Here's how the part is built. I have some questions about the finished solid (model axes, mm). Face numbers are marked on the shaded views. A direction names the side the tool comes from. Round coordinates to 2 decimals unless told otherwise and drop trailing zeros. Write each loop counter-clockwise with the first axis right and the second up, starting at its lowest first coordinate (ties: lowest second). Pieces come first, ordered by that corner, then holes. Notation, with made-up numbers: (20.5, -10) -> (47.5, -10) arc R7 ccw to (47.5, 0) -> close; hole circle Ø5 at (36, 36). An arc over 180 degrees is marked (long way). Answer as CSV lines item,"result".
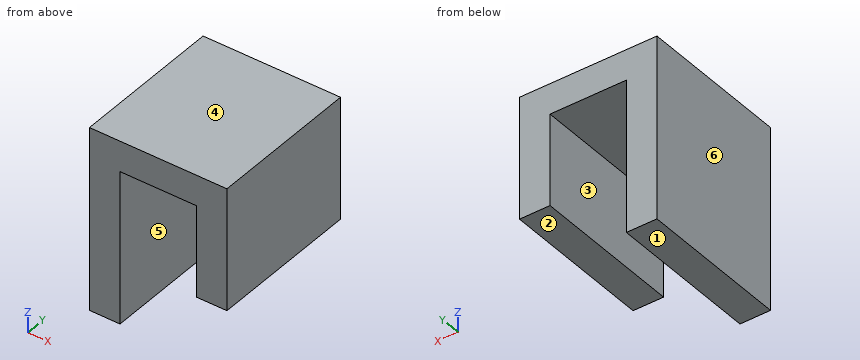
Autodesk Fusion 360 part; units mm, degrees
sketch "Sketch1" plane through (0, 0, 0) normal (0, 0, 1) x (1, 0, 0)
  line L0 (0, 0) -> (2, 0)
  line L1 (2, 0) -> (2, 10)
  line L2 (2, 10) -> (0, 10)
  line L3 (0, 10) -> (0, 0)
  dimension "d4" = 10
  dimension "d5" = 2
extrude "Extrude1" add sketch "Sketch1" along normal blind 12
sketch "Sketch2" plane through (2, 0, 0) normal (1, 0, 0) x (0, 1, 0)
  line L0 (0, 0) -> (10, 0)
  line L1 (10, 0) -> (10, 12)
  line L2 (10, 12) -> (0, 12)
  line L3 (0, 12) -> (0, 0)
  line L4 (0, 12) -> (10, 12)
  line L5 (10, 12) -> (10, 10)
  line L6 (10, 10) -> (0, 10)
  line L7 (0, 10) -> (0, 12)
  dimension "d8" = 2
extrude "Extrude2" add sketch "Sketch2" along normal blind 7 contours L1 L2 L3 L4 L5 L6 L7
sketch "Sketch3" plane through (0, 0, 10) normal (0, 0, -1) x (1, 0, 0)
  line L0 (2, 0) -> (2, -10)
  line L1 (2, -10) -> (9, -10)
  line L2 (9, -10) -> (9, 0)
  line L3 (9, 0) -> (2, 0)
  line L4 (9, -10) -> (7, -10)
  line L5 (7, -10) -> (7, 0)
  line L6 (7, 0) -> (9, 0)
  line L7 (9, 0) -> (9, -10)
  dimension "d11" = 2
extrude "Extrude3" add sketch "Sketch3" along normal blind 6 contours L1 L2 L3 L4 L5 L6 L7
equation "width = 10 mm"
equation "length = 2 mm"
equation "height = 12 mm"
equation "d4 = width"
equation "d5 = length"
equation "d6 = height"
Item 1: For the marked faces 1, 2 and 3, which set-ups out of +Z, -Z, +X, -X, +Y, -Y let a thin tool reach every point of the face, with its end or its side?
Results found:
face 1,"-Z, +X, -X, +Y, -Y"
face 2,"-Z, +X, +Y, -Y"
face 3,"-Z, +Y, -Y"
Item 2: Suppose I cut it at C-C, the plane z = 3. List the corners of the cut face in (x, y) for me.
Results found:
outline,"(0, 0) -> (2, 0) -> (2, 10) -> (0, 10) -> close"
Item 3: Suppose I cut it at A-A, the plane z = 5. List the corners of the cut face in (x, y) for me.
Results found:
outline,"(0, 0) -> (2, 0) -> (2, 10) -> (0, 10) -> close; (7, 0) -> (9, 0) -> (9, 10) -> (7, 10) -> close"
Item 4: Suppose I cut it at B-B, the plane y = 6.75. List the corners of the cut face in (x, z) for me, then the cut area to 3 significant figures.
Results found:
outline,"(0, 0) -> (2, 0) -> (2, 10) -> (7, 10) -> (7, 4) -> (9, 4) -> (9, 12) -> (0, 12) -> close"
area,"50.0 mm²"
Item 5: Suppose I cut it at D-D, the plane x = 8. List the corners of the cut face in (y, z) for me, then the cut area to 3 significant figures.
Results found:
outline,"(0, 4) -> (10, 4) -> (10, 12) -> (0, 12) -> close"
area,"80.0 mm²"
Item 6: I need wall thicknesses on L1, parallel to X at y = 7, z = 6.75; L2, parallel to Z at x = 3, y = 1.75; L3, parallel to X at y = 2.75, z = 2.75. Which ranges of each line are inside material? Lowest first, please.
Results found:
L1,"x = 0 to 2, 7 to 9"
L2,"z = 10 to 12"
L3,"x = 0 to 2"
Item 7: Will these pins go through, and if not, where does the flat tip stop? pin 1 (1.5 mm diameter, centred on x = 5.5, y = 6.5, fed in from -Z); pin 2 (1.5 mm diameter, centred on y = 7, z = 9, fed in from -X); pin 3 (2 mm diameter, centred on x = 8.5, y = 6, fed in from -Z); pin 4 (1.5 mm diameter, centred on y = 4.5, z = 3, fed in from +X).
Results found:
pin 1,"stops at z = 10"
pin 2,"stops at x = 0"
pin 3,"stops at z = 4"
pin 4,"stops at x = 2"
Item 8: If we mould it in two halves opening along X, with no side actions, what happens to the marked faces 4, 5 and 6? For each: pulls with the +X half, pulls with the -X half, needs draft (parallel to the pull), parting line crosses it, or undercut.
Results found:
face 4,"needs draft"
face 5,"undercut"
face 6,"pulls with the -X half"
